Work out the finished part from the listing and answer in its coordinate system (mm). Round coordinates to 2 decimals unless told otherwise and drop trailing zeros. Write each loop counter-clockwise with the first axis right and the second up, starting at its lowest first coordinate (ties: lowest second). Pieces come first, ordered by that corner, then holes.
1. Find section B-B (x = 5). Write down the section's boundary in (y, z).
2. Find section C-C (z = 35). Write down the section's boundary in (x, y), and give its area (3 significant figures).
3. Straight lines are drawn through the part: probe 1 along Z at (x, y) = (21.5, 12); probe 2 along Z at (x, y) = (19, 20); probe 3 along Y at (x, z) = (1.5, 66). For each, find the intervals that lie inside material, in ascending order.
4. Find section A-A (z = 14.5). Write down the section's boundary in (x, y).
5. Flat-ended cylindrical pins translate along their axes: pin 1 Ø8 at (x, z) = (-11.5, 48.5) entering from -Y; pin 2 Ø3 at (y, z) = (19, 36.5) entering from +X; pin 3 Ø3 at (y, z) = (20.5, 18.5) entering from -X; pin 4 Ø3 at (x, z) = (21, 68.5) entering from +Y. Find the tip coordinate at first contact, or state that the pin passes through.
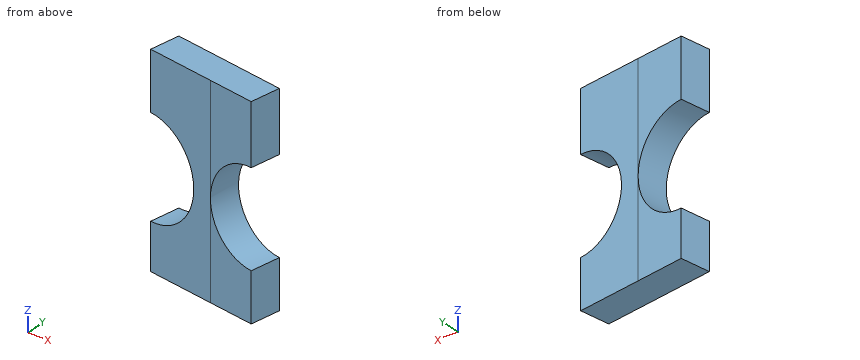
Autodesk Inventor part; units mm, degrees
ref_plane "Work Plane2" through (-150.8486, -254.8124, 77.677) normal (0, 0, -1) x (0, 1, 0)
ref_plane "YZ Plane" through (0, 0, 0) normal (1, 0, 0) x (0, 1, 0)
ref_plane "XZ Plane" through (0, 0, 0) normal (0, 1, 0) x (-1, 0, 0)
ref_plane "Work Plane1" through (0, 0, 0) normal (0, 0, 1) x (1, 0, 0)
sketch "Sketch1" plane through (0, 0, 0) normal (0, 0, 1) x (1, 0, 0)
  line L0 (46.9411, 24.4056) -> (43.9673, 4.6279) construction
  line L1 (-34.7264, 28.3648) -> (-39.7819, -5.2572) construction
  line L2 (9.0191, -106.7418) -> (35.6521, 70.3833) construction
  line L3 (-3.8449, 105.9638) -> (-30.4779, -71.1613) construction
  line L4 (8.3675, 9.9808) -> (26.1674, 7.3043)
  line L5 (8.3675, 9.9808) -> (-17.688, 13.8986)
  line L6 (2.8511, 22.7146) -> (27.9178, 18.9455)
  line L7 (2.8511, 22.7146) -> (-15.9376, 25.5397)
  line L8 (-15.9376, 25.5397) -> (-17.688, 13.8986)
  line L9 (27.9178, 18.9455) -> (26.1674, 7.3043)
  point P0 (0, 0)
ref_plane "Work Plane2" through (-150.8486, -254.8124, 77.677) normal (0, 0, -1) x (0, 1, 0)
extrude "Extrusion1" add sketch "Sketch1" along normal up to surface (77.677 mm away)
sketch "Sketch2" plane through (27.9178, 18.9455, 77.677) normal (0.1487, 0.9889, 0) x (0.9889, -0.1487, 0)
  circle A0 centre (0, 41.0877) radius 18 construction
  circle A1 centre (-44.3484, 41.0877) radius 19 construction
  circle A2 centre (-44.3484, 41.0877) radius 19
  circle A3 centre (0, 41.0877) radius 18
  point P0 (-24.7904, 77.677)
extrude "Extrusion2" cut sketch "Sketch2" against normal through all
properties part number "motor mount center"
Worked answers:
1. outline: (10.49, 0) - (22.39, 0) - (22.39, 77.68) - (10.49, 77.68) - close
2. outline: (1.03, 11.08) - (8.37, 9.98) - (8.44, 9.97) - (10.19, 21.61) - (2.85, 22.71) - (2.79, 22.72) - close
2. area: 88.1 mm2
3. probe 1: z = 0 to 19.39, 53.79 to 77.68
3. probe 2: z = 0 to 20.99, 52.19 to 77.68
3. probe 3: y = 11.01 to 22.92
4. outline: (-17.69, 13.9) - (8.37, 9.98) - (26.17, 7.3) - (27.92, 18.95) - (2.85, 22.71) - (-15.94, 25.54) - close
5. pin 1: passes through
5. pin 2: stops at x = 9.95
5. pin 3: stops at x = -16.87
5. pin 4: stops at y = 20.21
